Here's how the part is built. I have some questions about the finished solid (model axes, mm). A direction names the side the tool comes from. Round coordinates to 2 decimals unless told otherwise and drop trailing zeros. Order: outer loops, then holes, each group sorted by start corner. A loop starts at its lowest first (then second) coordinate and runs counter-clockwise, first axis right, second up. Notation, with made-up numbers: (52, -14) -> (109, -14) arc R17 ccw to (109, -5) -> close; hole circle Ø5 at (59.5, -29.5). An arc over 180 degrees is marked (long way). Use a Markdown table: item, result. Add a question column.
from build123d import *

# Parameters (mm, degrees)
SKETCH3_W                = 20
SKETCH3_H                = 12
BOSS_EXTRUDE3_DEPTH      = 2
BOSS_EXTRUDE5_DEPTH      = 20
BOSS_EXTRUDE5_DEPTH_BACK = 20
SKETCH4_W                = 20
SKETCH4_H                = 5
CUT_EXTRUDE1_DEPTH       = 20
SKETCH7_W                = 8.512199936
SKETCH7_H                = 1.761144814
SKETCH7_W_2              = 9.304715103
SKETCH7_H_2              = 2
CUT_EXTRUDE2_DEPTH       = 35.249087579


with BuildPart() as part:
    # Sketch3 → Boss-Extrude3 (new body)
    with BuildSketch(Plane(origin=(0, 0, 0), x_dir=(0, 0, -1), z_dir=(1, 0, 0))):
        with Locations((10, -6)):
            Rectangle(SKETCH3_W, SKETCH3_H)
    extrude(amount=BOSS_EXTRUDE3_DEPTH)

    # Sketch4 → Boss-Extrude5 (add, two sides: drawn at the far end of the back side and taken through both)
    with BuildSketch(Plane(origin=(2, 0, 0), x_dir=(0, 0, -1), z_dir=(1, 0, 0)).offset(-BOSS_EXTRUDE5_DEPTH_BACK)):
        with Locations((10, -14.5)):
            Rectangle(SKETCH4_W, SKETCH4_H)
    extrude(amount=BOSS_EXTRUDE5_DEPTH + BOSS_EXTRUDE5_DEPTH_BACK)

    # Sketch6 → Cut-Extrude1 (cut)
    with BuildSketch(Plane(origin=(22, 0, 0), x_dir=(0, 0, -1), z_dir=(1, 0, 0))):
        Polygon((7.5, -12), (12.5, -12), (15, -15.5), (5, -15.5), align=None)
    extrude(amount=-CUT_EXTRUDE1_DEPTH, mode=Mode.SUBTRACT)

    # Sketch7 → Cut-Extrude2 (cut, through all)
    with BuildSketch(Plane(origin=(0, 0, -20), x_dir=(-1, 0, 0), z_dir=(0, 0, -1))):
        with Locations((8.743900032, -14.380572407)):
            Rectangle(SKETCH7_W, SKETCH7_H)
        with Locations((-12.347642449, -14.5)):
            Rectangle(SKETCH7_W_2, SKETCH7_H_2)
    extrude(amount=-CUT_EXTRUDE2_DEPTH, mode=Mode.SUBTRACT)


solid = part.part
(1) Please list where these lines run through material, in increasing order: probe 1 along Y at (x, z) = (-7.5, -9.75); probe 2 along Y at (x, z) = (16, -14); probe 3 along X at (y, z) = (-9.75, -2.75). Write a range as from..to.
(2) If we mould it in two halves opening along Y, with no side actions, what happens to faces 5 (the flat face through (3.4, -12.3, -20)), 6 (the flat face through (-4.488, -14, -10)), 7 (the flat face through (-9, -12, -10))? For each: pulls with the +Y half, pulls with the -Y half, needs draft (parallel to the pull), parting line crosses it, or undercut.
(3) I want a section at D-D on z = -17.25. List the corners of the cut face in (x, y) for me.
(4) I want a section at C-C on z = -9.5. List the corners of the cut face in (x, y) for me, and give its area (3 significant figures).
(5) I want a section at A-A on x = -8.5. List the corners of the cut face in (y, z) for me.
(6) I'm going to push flat-ended pins straight in: P1, Ø1.5, axis at x = 4, y = -5, coming from the -Z side; P2, Ø2, axis at y = -5, z = -16, coming from the +X side; P3, Ø2.5, axis at x = -10.5, z = -15, coming from the +Y side; P4, Ø6, axis at y = -7, z = -8, coming from the -X side. Where does each tip first touch, or does it pass through?
(7) I want a section at B-B on y = -14. List the corners of the cut face in (x, z) for me.
(8) On a 3-axis mill with a long thin cutter (end or side, diameter ignored), from which of +Z, -Z, +X, -X, +Y, -Y can I reach the whole of each face in a straight line? I mean faces 1 (the flat face through (12, -12, -4)), 2 (the flat face through (-9, -13.5, -10)), 3 (the flat face through (0, -6, -10)), 4 (the flat face through (12, -15.5, -10)). Say none if no direction works.
Output:
| question | item | result |
|---|---|---|
| 1 | probe 1 | -17..-15.26, -13.5..-12 |
| 1 | probe 2 | -17..-15.5, -13.5..-12 |
| 1 | probe 3 | 0..2 |
| 2 | face 5 | needs draft |
| 2 | face 6 | undercut |
| 2 | face 7 | pulls with the +Y half |
| 3 | outline | (-18, -17) -> (22, -17) -> (22, -12) -> (2, -12) -> (2, 0) -> (0, 0) -> (0, -12) -> (-18, -12) -> close; hole (-13, -15.26) -> (-4.49, -15.26) -> (-4.49, -13.5) -> (-13, -13.5) -> close; hole (7.7, -15.5) -> (17, -15.5) -> (17, -13.5) -> (7.7, -13.5) -> close |
| 4 | outline | (-18, -17) -> (22, -17) -> (22, -15.5) -> (2, -15.5) -> (2, 0) -> (0, 0) -> (0, -12) -> (-18, -12) -> close; hole (-13, -15.26) -> (-4.49, -15.26) -> (-4.49, -13.5) -> (-13, -13.5) -> close |
| 4 | area | 139 mm² |
| 5 | outline | (-17, -20) -> (-15.26, -20) -> (-15.26, 0) -> (-17, 0) -> close; (-13.5, -20) -> (-12, -20) -> (-12, 0) -> (-13.5, 0) -> close |
| 6 | P1 | through |
| 6 | P2 | x = 2 |
| 6 | P3 | y = -12 |
| 6 | P4 | x = 0 |
| 7 | outline | (-18, -20) -> (-13, -20) -> (-13, 0) -> (-18, 0) -> close; (-4.49, -20) -> (7.7, -20) -> (7.7, -13.93) -> (2, -13.93) -> (2, -6.07) -> (7.7, -6.07) -> (7.7, 0) -> (-4.49, 0) -> close; (17, -20) -> (22, -20) -> (22, -13.93) -> (17, -13.93) -> close; (17, -6.07) -> (22, -6.07) -> (22, 0) -> (17, 0) -> close |
| 8 | face 1 | +Z, -Z, +X, +Y |
| 8 | face 2 | +Z, -Z |
| 8 | face 3 | +Z, -Z, -X, +Y |
| 8 | face 4 | none |
